CAD build for the part. Positions are in the model's coordinates, mm. Give positions to 0.01 mm unless a question says otherwise; leave off trailing zeros. Write each loop counter-clockwise with the first axis right and the second up, starting at its lowest first coordinate (ties: lowest second). Pieces come first, ordered by that corner, then holes. Notation, with made-up numbers: (22.5, 82.25) - (46.5, 82.25) arc R18 ccw to (46.5, 104.25) - close; hole circle Ø6 at (60.25, -1.5). An arc over 180 degrees is marked (long way). Answer as a JSON object with one key per item and string values.
from build123d import *

# Parameters (mm, degrees)
SKETCH1_R           = 2.65
SKETCH1_R_2         = 0.65
BOSS_EXTRUDE1_DEPTH = 1


with BuildPart() as part:
    # Sketch1 → Boss-Extrude1 (new body)
    with BuildSketch(Plane.ZY.offset(-16.004809472)):
        with BuildLine():
            Line((43.488619522, 61.406385053), (10.382219934, 114.514122983))
            ThreePointArc((10.382219934, 114.514122983), (6.429799658, 119.354410747), (9.035439795, 113.674564697))
            Line((9.035439795, 113.674564697), (42.141839383, 60.566826767))
            ThreePointArc((42.141839383, 60.566826767), (44.282136198, 58.633462713), (43.488619522, 61.406385053))
        make_face()
        with Locations((8.096184677, 116.681273832)):
            Circle(SKETCH1_R, mode=Mode.SUBTRACT)
        with Locations((43.488619522, 59.906385053)):
            Circle(SKETCH1_R_2, mode=Mode.SUBTRACT)
    extrude(amount=BOSS_EXTRUDE1_DEPTH)


solid = part.part
Item 1: Mould opens along Z. For faces 1 (the cylindrical face through (15.512, 59.511, 42.973)), 2 (the flat face through (15.005, 89, 25)), 3 (the cylindrical face through (15.51, 58.61, 44.24)), 4 (the flat face through (15.512, 87.588, 27.167)) say: +Z half, -Z half, draft (parallel to the pull), parting line (faces both ways), or undercut.
Entries:
{"face 1": "undercut", "face 2": "draft", "face 3": "parting line", "face 4": "+Z half"}
Item 2: Cut at B-B (y = 66). Give the cut face in (x, z).
Entries:
{"outline": "(15, 38.75) - (16, 38.75) - (16, 40.63) - (15, 40.63) - close"}
Item 3: Cut at C-C (z = 41). Give the cut face in (x, y), and give its area (3 significant figures).
Entries:
{"outline": "(15, 62.4) - (16, 62.4) - (16, 65.4) - (15, 65.4) - close", "area": "3.00 mm2"}
Item 4: Probe line 1 (Y direction, x = 15.85, z = 10); line 2 (Y direction, x = 15.6, z = 9); line 3 (Z direction, x = 15.8, y = 109.5). List the from-to ranges inside material, lowest first. Write a range as from..to.
Entries:
{"line 1": "112.13..114.84, 118.52..119.19", "line 2": "113.66..114.19, 119.17..119.7", "line 3": "11.64..13.51"}
Item 5: Cut at A-A (x = 15.8). Give the cut face in (y, z), and give its area (3 significant figures).
Entries:
{"outline": "(60.57, 42.14) - (113.67, 9.04) arc R3.15 ccw (long way) to (114.51, 10.38) - (61.41, 43.49) arc R1.5 ccw (long way) to start; hole circle Ø1.3 at (59.91, 43.49); hole circle Ø5.3 at (116.68, 8.1)", "area": "114 mm2"}
